Could you check a few things on this model? Use its own coordinates, in mm. A direction names the side the tool comes from. Round coordinates to 2 decimals unless told otherwise and drop trailing zeros. Write each loop counter-clockwise with the first axis right and the second up, starting at its lowest first coordinate (ties: lowest second). Pieces come first, ordered by that corner, then holes. Notation, with made-up numbers: (88.25, 17) - (104.25, 17) arc R24 ccw to (104.25, 39) - close; hole circle Ø11 at (-36.75, 84). An arc over 180 degrees is marked (long way). Write each question's results on one line, items separated by ' | '. Start each with the question number.
(1) Imagine slicing it at D-D on y = 1. Write out the boundary of the cut face in (x, z) (3 decimals).
(2) Imagine slicing it at C-C on z = 1.5. Write out the boundary of the cut face in (x, y) (3 decimals).
(3) Imagine slicing it at A-A on x = -4.25. Write out the boundary of the cut face in (y, z), then the cut area to 3 significant figures.
(4) For P1, Ø3, axis at x = -6.35, y = 3.175, coming from the +Z side; P2, Ø1.5, axis at y = 2, z = 1.5, coming from the -X side; P3, Ø3, axis at x = 4, y = 3, coming from the +Z side, each with a flat end and sliding along its axis, tell me the tip position at first contact or that it passes through.
(5) Thinking about a two-plate mould opening in Y: for faces 1 (the flat face through (-5, 3, 2.375)), 2 (the cylindrical face through (-9.524, 3.105, 1.171)), 3 (the flat face through (-3, 0, 3)), 4 (the cylindrical face through (-5.27, 3.51, 1.2)), which applies, +Y half, -Y half, draft (parallel to the pull), parting line (faces both ways), or undercut?
(6) Imagine slicing it at B-B on x = -7.25. Write out the boundary of the cut face in (y, z).
(7) Please list where these lines run through material, in increasing order: line 1 (Z direction, x = -8.25, y = 3.25); line 2 (Y direction, x = -6.35, z = 5.3); line 3 (X direction, y = 3.25, z = 5.5). Write a range as [from, to].
(8) On a 3-axis mill with a long thin cutter (end or side, diameter ignored), from which of +Z, -Z, +X, -X, +Y, -Y can I reach the whole of each face in a straight line? I mean faces 5 (the cylindrical face through (-5.497, 4.514, 5.179)), 6 (the flat face through (0, 5, 1)), 7 (the flat face through (-3.175, 1, 3)). Say none if no direction works.
```python
from build123d import *

# Parameters (mm, degrees)
BOSS_EXTRUDE1_DEPTH           = 6.35
SKETCH2_R                     = 2.5781
BOSS_EXTRUDE2_DEPTH           = 6.35
TAP_DRILL_FOR_6_32_TAP1_D     = 2.7051
TAP_DRILL_FOR_6_32_TAP1_DEPTH = 9.525
TAP_DRILL_FOR_6_32_TAP1_TIP   = 0.81269403
CUT_EXTRUDE1_REACH            = 15.091
SKETCH5_W                     = 10.16
SKETCH5_H                     = 1.6002
CUT_EXTRUDE2_REACH            = 15.091
SKETCH6_R                     = 1.5875
F_4_40_TAPPED_HOLE1_D         = 2.2606


with BuildPart() as part:
    # Sketch1 → Boss-Extrude1 (new body)
    with BuildSketch(Plane.XY):
        with BuildLine():
            Line((0, 0), (-6.35, 0))
            ThreePointArc((-6.35, 0), (-9.525, 3.175), (-6.35, 6.35))
            Line((-6.35, 6.35), (0, 6.35))
            Line((0, 6.35), (0, 0))
        make_face()
    extrude(amount=BOSS_EXTRUDE1_DEPTH)

    # Sketch2 → Boss-Extrude2 (add)
    with BuildSketch(Plane(origin=(0, 0, 0), x_dir=(0, 0, -1), z_dir=(1, 0, 0))):
        with Locations((-3.175, 3.175)):
            Circle(SKETCH2_R)
    extrude(amount=BOSS_EXTRUDE2_DEPTH)

    # Tap Drill for #6-32 Tap1
    with Locations(Plane(origin=(6.35, 0, 0), x_dir=(0, 0, -1), z_dir=(1, 0, 0))):
        with Locations((-3.175, 3.175)):
            Hole(TAP_DRILL_FOR_6_32_TAP1_D / 2, depth=TAP_DRILL_FOR_6_32_TAP1_DEPTH)
            with Locations((0, 0, -(TAP_DRILL_FOR_6_32_TAP1_DEPTH + TAP_DRILL_FOR_6_32_TAP1_TIP / 2))):  # 118° drill point
                Cone(0, TAP_DRILL_FOR_6_32_TAP1_D / 2, TAP_DRILL_FOR_6_32_TAP1_TIP, mode=Mode.SUBTRACT)

    # Sketch5 → Cut-Extrude1 (cut, up to next)
    with BuildSketch(Plane.XZ, mode=Mode.PRIVATE) as cut_extrude1_sk1:
        with Locations((-8.255, 3.175)):
            Rectangle(SKETCH5_W, SKETCH5_H)
    cut_extrude1_tool1 = extrude(cut_extrude1_sk1.sketch, amount=-CUT_EXTRUDE1_REACH, mode=Mode.PRIVATE) & part.part
    add(cut_extrude1_tool1.solids().sort_by_distance((-8.255, 0, 3.175))[0], mode=Mode.SUBTRACT)

    # Sketch6 → Cut-Extrude2 (cut, up to next)
    with BuildSketch(Plane.XY.offset(6.35), mode=Mode.PRIVATE) as cut_extrude2_sk1:
        with Locations((-6.35, 3.175)):
            Circle(SKETCH6_R)
    cut_extrude2_tool1 = extrude(cut_extrude2_sk1.sketch, amount=-CUT_EXTRUDE2_REACH, mode=Mode.PRIVATE) & part.part
    add(cut_extrude2_tool1.solids().sort_by_distance((-6.35, 3.175, 6.35))[0], mode=Mode.SUBTRACT)

    # #4-40 Tapped Hole1 (through all)
    with Locations(Plane(origin=(0, 0, 0), x_dir=(-1, 0, 0), z_dir=(0, 0, -1))):
        with Locations((6.35, 3.175)):
            Hole(F_4_40_TAPPED_HOLE1_D / 2)


solid = part.part
```
Response:
1) outline: (-8.663, 0) - (0, 0) - (0, 1.791) - (6.35, 1.791) - (6.35, 4.559) - (0, 4.559) - (0, 6.35) - (-8.663, 6.35) - (-8.663, 3.975) - (-3.175, 3.975) - (-3.175, 2.375) - (-8.663, 2.375) - close
2) outline: (-6.35, 0) - (0, 0) - (0, 1.215) - (6.35, 1.215) - (6.35, 5.135) - (0, 5.135) - (0, 6.35) - (-6.35, 6.35) arc R3.175 ccw to start; hole circle Ø2.261 at (-6.35, 3.175)
3) outline: (0, 0) - (6.35, 0) - (6.35, 2.37) - (0, 2.37) - close; (0, 3.98) - (6.35, 3.98) - (6.35, 6.35) - (0, 6.35) - close | area: 30.2 mm²
4) P1: z = 2.37 | P2: x = -9.5 | P3: z = 5.75
5) face 1: draft | face 2: parting line | face 3: -Y half | face 4: undercut
6) outline: (0.13, 0) - (2.49, 0) - (2.49, 2.37) - (0.13, 2.37) - close; (0.13, 3.98) - (1.87, 3.98) - (1.87, 6.35) - (0.13, 6.35) - close; (3.86, 0) - (6.22, 0) - (6.22, 2.37) - (3.86, 2.37) - close; (4.48, 3.98) - (6.22, 3.98) - (6.22, 6.35) - (4.48, 6.35) - close
7) line 1: [0, 2.37], [3.98, 6.35] | line 2: [0, 1.59], [4.76, 6.35] | line 3: [-9.52, -7.94], [-4.76, 6.35]
8) face 5: +Z | face 6: +X | face 7: -X, +Y, -Y
